The model under review builds one solid part; all positions refer to its coordinate system, in mm. A direction names the side the tool comes from. Coordinates: 2 decimals unless noted, no trailing zeros. Order: outer loops, then holes, each group sorted by start corner. A loop starts at its lowest first (then second) coordinate and runs counter-clockwise, first axis right, second up. Notation, with made-up numbers: (-19.5, -12.5) -> (15.5, -12.5) arc R4 cw to (15.5, -7.5) -> close; hole circle Ø1 at (3, 36.5). An arc over 180 degrees is marked (long way). Use CSV: the item, a comma, the result in double quotes. Start each with the question number.
```python
from build123d import *

# Parameters (mm, degrees)
F2_R     = 7.5
F3_DEPTH = 33


with BuildPart() as f1:
    # F0 (on Right) → F1 (revolve)
    with BuildSketch(Plane.YZ):
        with BuildLine():
            Line((3, 32), (3, 0))
            Line((3, 0), (21, 0))
            Line((21, 0), (21, 26))
            Line((21, 26), (63, 26))
            Line((63, 26), (63, 29))
            Line((63, 29), (93, 31))
            Line((93, 31), (93, 39))
            Line((93, 39), (85, 39))
            Line((85, 39), (85, 45))
            Line((85, 45), (55, 45))
            Line((55, 45), (55, 33.200345))
            ThreePointArc((55, 33.200345), (52.308743, 28.765291), (47.132118, 29.104585))
            Line((47.132118, 29.104585), (33, 39))
            Line((33, 39), (0, 39))
            Line((0, 39), (0, 32))
            Line((0, 32), (3, 32))
        make_face()
    revolve(axis=Axis((0, 12, 0), (0, -1, 0)))

    # F2 (on Front) → F3 (join)
    with BuildSketch(Plane.XZ):
        with BuildLine():
            Line((37.494811, 10.730289), (18.266703, 77.918999))
            ThreePointArc((18.266703, 77.918999), (0, 91.691422), (-18.266703, 77.918999))
            Line((-18.266703, 77.918999), (-37.494811, 10.730289))
            ThreePointArc((-37.494811, 10.730289), (0, 39), (37.494811, 10.730289))
        make_face()
        with Locations((0, 72.691422)):
            Circle(F2_R, mode=Mode.SUBTRACT)
        with BuildLine():
            ThreePointArc((37.494811, -10.730289), (0, -39), (-37.494811, -10.730289))
            Line((-37.494811, -10.730289), (-18.266703, -77.918999))
            ThreePointArc((-18.266703, -77.918999), (0, -91.691422), (18.266703, -77.918999))
            Line((18.266703, -77.918999), (37.494811, -10.730289))
        make_face()
        with Locations((0, -72.691422)):
            Circle(F2_R, mode=Mode.SUBTRACT)
    extrude(amount=-F3_DEPTH)


solid = f1.part
```
Q1. Add section C-C, the plane y = 24.5. State the section outline as (x, z) points, then the cut area to 3 significant figures.
Q2. To check wall thickness, follow probe 1 along Z at (x, y) = (0, 13); probe 2 along Z at (x, y) = (0, 24.5); probe 3 along Z at (x, y) = (0, 1.55). State the ranges of each line that lie inside material, in increasing order.
Q3. For faces 1 (the flat face through (27.746, 16.269, -44.795)), 2 (the flat face through (28.015, 16.269, 43.854)), 3 (the conical face through (-8.93, 46.25, 28.35)), 4 (the flat face through (0, 3, 0)), list the 3-axis set-ups (+Z, -Z, +X, -X, +Y, -Y) from which the entire face can be reached by the end or side of a thin tool; tool diameter is ignored.
Q4. Clearance check with flat-ended pins moving along their axes: pin 1 Ø3 at (x, y) = (28.5, 37.5) entering from -Z; pin 2 Ø12 at (x, z) = (0, 72.69) entering from -Y; pin 3 Ø2 at (x, y) = (4.5, 65) entering from -Z; pin 4 Ø12 at (x, z) = (18.5, 68) entering from +Y. State where each tip first meets the part, or that it passes through.
Q5. Draft analysis for pull direction X (two halves, no side actions). For faces 5 (the flat face through (-24, 63, 11)), 6 (the flat face through (-37, 85, 14)), 7 (the cylindrical face through (39, 16, 0)), 8 (the cylindrical face through (0.34, 16.27, 91.69)), state which applies: +X half, -X half, draft (parallel to the pull), parting line (faces both ways), or undercut.
Q6. Add section A-A, the plane z = 0. State the section outline as (x, y) points, then the cut area to 3 significant figures.
Q7. Add section D-D, the plane x = 0. State how many separate pieces and enclosed holes the cut face has, then the cut area to 3 significant figures.
Q8. Add section B-B, the plane y = 60. State the section outline as (x, z) points.
Answer block:
1,outline,"(-37.49, -10.73) -> (-18.27, -77.92) arc R19 ccw to (18.27, -77.92) -> (37.49, -10.73) arc R39 ccw to (37.49, 10.73) -> (18.27, 77.92) arc R19 ccw to (-18.27, 77.92) -> (-37.49, 10.73) arc R39 ccw to start; hole circle Ø52 at (0, 0); hole circle Ø15 at (0, -72.69); hole circle Ø15 at (0, 72.69)"
1,area,"7,410 mm²"
2,probe 1,"z = -91.69 to -80.19, -65.19 to 65.19, 80.19 to 91.69"
2,probe 2,"z = -91.69 to -80.19, -65.19 to -26, 26 to 65.19, 80.19 to 91.69"
2,probe 3,"z = -91.69 to -80.19, -65.19 to -32, 32 to 65.19, 80.19 to 91.69"
3,face 1,"-Z, +X, -Y"
3,face 2,"+Z, +X, -Y"
3,face 3,"none"
3,face 4,"-Y"
4,pin 1,"stops at z = -24.21"
4,pin 2,"passes through"
4,pin 3,"stops at z = -44.86"
4,pin 4,"stops at y = 33"
5,face 5,"undercut"
5,face 6,"draft"
5,face 7,"+X half"
5,face 8,"parting line"
6,outline,"(-45, 55) -> (-33.2, 55) arc R5 cw to (-29.1, 47.13) -> (-39, 33) -> (-39, 0) -> (-32, 0) -> (-32, 3) -> (32, 3) -> (32, 0) -> (39, 0) -> (39, 33) -> (29.1, 47.13) arc R5 cw to (33.2, 55) -> (45, 55) -> (45, 85) -> (39, 85) -> (39, 93) -> (31, 93) -> (29, 63) -> (26, 63) -> (26, 21) -> (-26, 21) -> (-26, 63) -> (-29, 63) -> (-31, 93) -> (-39, 93) -> (-39, 85) -> (-45, 85) -> close"
6,area,"3,140 mm²"
7,separate pieces,"3"
7,enclosed holes,"0"
7,area,"5,630 mm²"
8,outline,"circle Ø90 at (0, 0); hole circle Ø52 at (0, 0)"
